Autodesk Inventor part; units mm, degrees
ref_plane "Work Plane1" through (-56.3599, 0, 22) normal (0, 0, -1) x (-1, 0, 0)
ref_plane "YZ Plane" through (0, 0, 0) normal (1, 0, 0) x (0, 1, 0)
ref_plane "XZ Plane" through (0, 0, 0) normal (0, 1, 0) x (-1, 0, 0)
ref_plane "Work Plane1" through (-56.3599, 0, 22) normal (0, 0, -1) x (-1, 0, 0)
sketch "Sketch1" plane through (-56.3599, 0, 22) normal (0, 0, -1) x (-1, 0, 0)
  line L0 (-4.0299, -0.3538) -> (-2.2322, 1.4439) construction
  arc A0 (-1.4439, 2.2322) -> (-2.2322, 1.4439) centre (-0.9299, 0.9299) ccw construction
  line L1 (-1.4439, 2.2322) -> (0.3538, 4.0299) construction
  line L2 (-37.8299, 42.8299) -> (-37.8299, 37.8299) construction
  line L3 (-37.8299, 37.8299) -> (-42.9208, 37.8299) construction
  line L4 (-37.8299, 42.2137) -> (-37.8299, 45.8299) construction
  line L5 (-37.8299, 45.8299) -> (-4.0299, 45.8299) construction
  line L6 (-4.0299, 45.8299) -> (-4.0299, 42.2137) construction
  line L7 (-4.0299, 4.0299) -> (0.3538, 4.0299)
  circle A1 centre (-20.9299, 20.9299) radius 17.5
  line L8 (-20.9299, 58.9723) -> (17.1124, 20.9299) construction
  line L9 (17.1124, 20.9299) -> (-20.9299, -17.1124) construction
  line L10 (-20.9299, -17.1124) -> (-58.9723, 20.9299) construction
  line L11 (-58.9723, 20.9299) -> (-20.9299, 58.9723) construction
  line L12 (-20.9299, 58.9723) -> (-20.9299, -17.1124) construction
  line L13 (17.1124, 20.9299) -> (-58.9723, 20.9299) construction
  line L14 (-20.9299, 58.9723) -> (32.8701, 58.9723) construction
  line L15 (-43.4299, 43.4299) -> (1.5701, 43.4299) construction
  line L16 (1.5701, 43.4299) -> (1.5701, -1.5701) construction
  line L17 (1.5701, -1.5701) -> (-43.4299, -1.5701) construction
  line L18 (-43.4299, -1.5701) -> (-43.4299, 43.4299) construction
  line L19 (-43.4299, 43.4299) -> (1.5701, -1.5701) construction
  line L20 (1.5701, 43.4299) -> (-43.4299, -1.5701) construction
  line L21 (-43.4299, 5.3876) -> (-43.4299, 36.4723)
  line L22 (-43.4299, 36.4723) -> (-36.4723, 43.4299)
  line L23 (-36.4723, 43.4299) -> (-5.3876, 43.4299)
  line L24 (-5.3876, 43.4299) -> (1.5701, 36.4723)
  line L25 (1.5701, 36.4723) -> (1.5701, 5.3876)
  line L26 (1.5701, 5.3876) -> (-5.3876, -1.5701)
  line L27 (-5.3876, -1.5701) -> (-36.4723, -1.5701)
  line L28 (-36.4723, -1.5701) -> (-43.4299, 5.3876)
  line L29 (-4.0299, 42.2137) -> (-37.8299, 42.2137)
  line L30 (-4.0299, -0.3538) -> (-4.0299, 4.0299)
  circle A2 centre (-20.9299, 20.9299) radius 1.5
  line L31 (-10.9299, 10.9299) -> (-30.9299, 10.9299) construction
  line L32 (-30.9299, 10.9299) -> (-30.9299, 30.9299) construction
  line L33 (-30.9299, 30.9299) -> (-10.9299, 30.9299) construction
  line L34 (-10.9299, 30.9299) -> (-10.9299, 10.9299) construction
  line L35 (-10.9299, 10.9299) -> (-30.9299, 30.9299) construction
  line L36 (-30.9299, 10.9299) -> (-10.9299, 30.9299) construction
  circle A3 centre (-30.9299, 30.9299) radius 1.4
  circle A4 centre (-30.9299, 10.9299) radius 1.4
  circle A5 centre (-10.9299, 10.9299) radius 1.4
  line L37 (-45.8299, 37.8299) -> (-42.0723, 37.8299) construction
  line L38 (-42.1723, 37.7299) -> (-45.8299, 37.7299)
  line L39 (-45.8299, 37.7299) -> (-45.8299, 4.1299)
  line L40 (-45.8299, 4.1299) -> (-42.1723, 4.1299)
  line L41 (-42.1723, 4.1299) -> (-42.1723, 37.7299)
  line L42 (-45.8299, 4.0299) -> (-42.0723, 4.0299) construction
  line L43 (-45.8299, 37.8299) -> (-42.0723, 37.8299)
  line L44 (-37.7299, 45.8299) -> (-4.1299, 45.8299)
  line L45 (-4.1299, 45.8299) -> (-4.1299, 42.1723)
  line L46 (-4.1299, 42.1723) -> (-37.7299, 42.1723)
  line L47 (-37.7299, 42.1723) -> (-37.7299, 45.8299)
  line L48 (0.4701, 37.8299) -> (0.4701, 4.0299) construction
  line L49 (0.4701, 4.0299) -> (3.9701, 4.0299) construction
  line L50 (3.9701, 37.8299) -> (3.9701, 4.0299) construction
  line L51 (0.4701, 37.8299) -> (3.9701, 37.8299) construction
  line L52 (-45.8299, -3.9701) -> (-4.0299, -3.9701) construction
  line L53 (0.3124, 37.7299) -> (3.9701, 37.7299)
  line L54 (3.9701, 37.7299) -> (3.9701, 4.1299)
  line L55 (3.9701, 4.1299) -> (0.3124, 4.1299)
  line L56 (0.3124, 4.1299) -> (0.3124, 37.7299)
  line L57 (-4.1713, -0.3538) -> (-37.7299, -0.3538)
  line L58 (-37.7299, -0.3538) -> (-37.7299, -3.9701)
  line L59 (-37.7299, -3.9701) -> (-4.1713, -3.9701)
  line L60 (-4.1713, -3.9701) -> (-4.1713, -0.3538)
  point P0 (-37.8299, 4.0299)
  dimension "d18" = 53.8
  dimension "d19" = 45
  dimension "d20" = 53.8
  dimension "d21" = 45
  dimension "d22" = 45
  dimension "d30" = 20
  dimension "d31" = 20
  dimension "d32" = 2.8
  dimension "d33" = 2.8
  dimension "d34" = 2.8
  dimension "d35" = 3
  dimension "d36" = 0.1
  dimension "d37" = 0.1
  dimension "d38" = 0.1
  dimension "d39" = 0.1
extrude "Extrusion1" add sketch "Sketch1" along normal blind 8 contours L30 L26 L57 L28 L41 L22 L46 L24 L56 L7 | L7 L26 L30 | L56 L24 L25 L26 | L26 L25 L24 L53 L54 L55 | L60 L59 L58 L57 L28 L27 L26 | L26 L27 L28 L57 | L46 L22 L29 L24 | L24 L29 L45 | L40 L39 L38 L22 L21 L28 | L28 L21 L22 L41 | L29 L22 L23 L24 | L24 L23 L22 L29 L47 L44 L45 | L47 L29 L22 | A1 | A2 | A3 | A4 | A5
sketch "Skizze4" plane through (-56.3599, 0, 14) normal (0, 0, -1) x (-1, 0, 0)
  line L0 (-37.7299, 42.1723) -> (-42.1723, 37.7299)
  line L1 (-42.1723, 37.7299) -> (-45.8299, 37.7299)
  line L2 (-45.8299, 37.7299) -> (-45.8299, 4.1299) construction
  line L3 (-45.8299, 4.1299) -> (-42.1723, 4.1299)
  line L4 (-42.1723, 4.1299) -> (-37.6885, -0.3538)
  line L5 (-37.6885, -0.3538) -> (-37.7299, -0.3538)
  line L6 (-37.7299, -0.3538) -> (-37.7299, -3.9701)
  line L7 (-37.7299, -3.9701) -> (-4.1713, -3.9701) construction
  line L8 (-4.1713, -3.9701) -> (-4.1713, -0.3538)
  line L9 (-4.1713, -0.3538) -> (0.3124, 4.1299)
  line L10 (0.3124, 4.1299) -> (3.9701, 4.1299)
  line L11 (3.9701, 4.1299) -> (3.9701, 37.7299) construction
  line L12 (3.9701, 37.7299) -> (0.3124, 37.7299)
  line L13 (0.3124, 37.7299) -> (-4.1299, 42.1723)
  line L14 (-4.1299, 42.1723) -> (-4.1299, 45.8299)
  line L15 (-4.1299, 45.8299) -> (-37.7299, 45.8299) construction
  line L16 (-37.7299, 45.8299) -> (-37.7299, 42.1723)
  line L17 (-37.9299, 46.0299) -> (-3.9299, 46.0299) construction
  line L18 (-3.9299, 46.0299) -> (-3.9299, 42.2551)
  line L19 (-3.9299, 42.2551) -> (0.3953, 37.9299)
  line L20 (0.3953, 37.9299) -> (4.1701, 37.9299)
  line L21 (4.1701, 37.9299) -> (4.1701, 3.9299) construction
  line L22 (4.1701, 3.9299) -> (0.3953, 3.9299)
  line L23 (0.3953, 3.9299) -> (-3.9713, -0.4367)
  line L24 (-3.9713, -0.4367) -> (-3.9713, -4.1701)
  line L25 (-3.9713, -4.1701) -> (-37.9299, -4.1701) construction
  line L26 (-37.9299, -4.1701) -> (-37.9299, -0.3953)
  line L27 (-37.9299, -0.3953) -> (-42.2551, 3.9299)
  line L28 (-42.2551, 3.9299) -> (-46.0299, 3.9299)
  line L29 (-46.0299, 3.9299) -> (-46.0299, 37.9299) construction
  line L30 (-46.0299, 37.9299) -> (-42.2551, 37.9299)
  line L31 (-42.2551, 37.9299) -> (-37.9299, 42.2551)
  line L32 (-37.9299, 42.2551) -> (-37.9299, 46.0299)
  line L33 (-45.8299, 37.7299) -> (-45.8299, 37.9299)
  line L34 (-4.1299, 45.8299) -> (-37.7299, 45.8299)
  line L35 (-37.7299, 45.8299) -> (-37.9299, 45.8299)
  line L36 (-4.1299, 45.8299) -> (-3.9299, 45.8299)
  line L37 (3.9701, 37.7299) -> (3.9701, 37.9299)
  line L38 (3.9701, 4.1299) -> (3.9701, 37.7299)
  line L39 (3.9701, 4.1299) -> (3.9701, 3.9299)
  line L40 (-4.1713, -3.9701) -> (-3.9713, -3.9701)
  line L41 (-37.7299, -3.9701) -> (-37.9299, -3.9701)
  line L42 (-45.8299, 4.1299) -> (-45.8299, 3.9299)
  point P0 (-56.3599, 0)
  dimension "d40" = 0.2
extrude "IM_offset" add sketch "Skizze4" against normal up to surface (8 mm away)
ref_plane "Arbeitsebene5" through (-35.4299, 3.9299, 22) normal (-1, 0, 0) x (0, 0, 1)
ref_plane "Arbeitsebene6" through (-18.4299, 20.9299, 22) normal (0, 1, 0) x (-1, 0, 0)
sketch "Skizze31" plane through (-56.3599, 0, 22) normal (0, 0, 1) x (1, 0, 0)
  line L0 (25.9049, 44.8899) -> (15.7949, 44.8899)
  spline S0 degree 3 poles (21.2744, 21.9194) (21.3357, 21.9462) (21.3936, 21.9718) (21.5033, 22.0154) (21.5491, 22.0289) (21.5827, 22.0289) (21.5892, 22.0276) (21.5935, 22.0247) knots 0.300335 0.300335 0.300335 0.300335 0.323424 0.323424 0.35266 0.35266 0.362351 0.362351 0.362351 0.362351
  line L1 (21.2744, 21.9194) -> (21.2744, 26.3899)
  line L2 (20.4254, 21.9194) -> (20.4254, 26.3899)
  line L3 (21.9714, 15.3899) -> (21.1087, 15.3899)
  line L4 (20.5911, 15.3899) -> (19.7285, 15.3899)
  line L5 (20.5999, 15.3899) -> (21.0999, 15.3899)
  line L6 (28.5999, 22.8289) -> (28.5999, 24.3299)
  line L7 (28.5999, 24.3299) -> (28.0999, 24.3299)
  line L8 (28.0999, 24.3299) -> (28.0999, 22.8289)
  line L9 (28.0999, 22.8289) -> (27.7114, 24.2788)
  line L10 (27.7114, 24.2788) -> (27.2285, 24.1494)
  line L11 (27.2285, 24.1494) -> (28.0911, 20.9299)
  line L12 (28.0911, 20.9299) -> (27.2285, 17.7105)
  line L13 (27.2285, 17.7105) -> (27.7114, 17.5811)
  line L14 (27.7114, 17.5811) -> (28.0999, 19.031)
  line L15 (28.0999, 19.031) -> (28.0999, 17.5299)
  line L16 (28.0999, 17.5299) -> (28.5999, 17.5299)
  line L17 (28.5999, 17.5299) -> (28.5999, 19.031)
  line L18 (28.5999, 19.031) -> (28.9884, 17.5811)
  line L19 (28.9884, 17.5811) -> (29.4714, 17.7105)
  line L20 (29.4714, 17.7105) -> (28.6087, 20.9299)
  line L21 (28.6087, 20.9299) -> (29.4714, 24.1494)
  line L22 (29.4714, 24.1494) -> (28.9884, 24.2788)
  line L23 (28.9884, 24.2788) -> (28.5999, 22.8289)
  circle A0 centre (28.3499, 20.9299) radius 1.35
  line L24 (3.9713, -3.9701) -> (37.9299, -3.9701)
  line L25 (37.9299, -3.9701) -> (37.9299, -0.3953)
  line L26 (37.9299, -0.3953) -> (42.2551, 3.9299)
  line L27 (42.2551, 3.9299) -> (45.8299, 3.9299)
  line L28 (45.8299, 3.9299) -> (45.8299, 37.9299)
  line L29 (45.8299, 37.9299) -> (42.2551, 37.9299)
  line L30 (42.2551, 37.9299) -> (37.9299, 42.2551)
  line L31 (37.9299, 42.2551) -> (37.9299, 45.8299)
  line L32 (37.9299, 45.8299) -> (3.9299, 45.8299)
  line L33 (3.9299, 45.8299) -> (3.9299, 42.2551)
  line L34 (3.9299, 42.2551) -> (-0.3953, 37.9299)
  line L35 (-0.3953, 37.9299) -> (-3.9701, 37.9299)
  line L36 (-3.9701, 37.9299) -> (-3.9701, 3.9299)
  line L37 (-3.9701, 3.9299) -> (-0.3953, 3.9299)
  line L38 (-0.3953, 3.9299) -> (3.9713, -0.4367)
  line L39 (3.9713, -0.4367) -> (3.9713, -3.9701)
  line L40 (45.8299, 37.9299) -> (45.8299, 3.9299)
  line L41 (20.8299, 20.4299) -> (45.8299, 20.4299)
  line L42 (45.8299, 20.4299) -> (45.8299, 21.4299)
  line L43 (45.8299, 21.4299) -> (20.8299, 21.4299)
  line L44 (20.8299, 21.4299) -> (20.8299, 20.4299)
  line L45 (20.8299, 20.4299) -> (45.8299, 21.4299) construction
  line L46 (45.8299, 20.4299) -> (20.8299, 21.4299) construction
  line L47 (45.8299, 30.4299) -> (20.8299, 30.4299)
  line L48 (20.8299, 30.4299) -> (20.8299, 27.4299)
  line L49 (20.8299, 27.4299) -> (45.8299, 27.4299)
  line L50 (45.8299, 27.4299) -> (45.8299, 30.4299)
  line L51 (45.8299, 14.4299) -> (20.8299, 14.4299)
  line L52 (20.8299, 14.4299) -> (20.8299, 11.4299)
  line L53 (20.8299, 11.4299) -> (45.8299, 11.4299)
  line L54 (45.8299, 11.4299) -> (45.8299, 14.4299)
  circle A1 centre (20.8299, 20.9299) radius 1.5
  point P0 (56.3599, 0)
  point P1 (33.3299, 20.9299)
  point P2 (45.8299, 11.4299)
  point P3 (27.0959, 20.4299)
  point P4 (29.6039, 20.4299)
  point P5 (29.6039, 21.4299)
  point P6 (27.0959, 21.4299)
  point P7 (22.2441, 21.4299)
  point P8 (22.2441, 20.4299)
  point P9 (45.8299, 27.4299)
  dimension "d181" = 2.7
  dimension "d182" = 1
  dimension "d183" = 3
  dimension "d184" = 3
  dimension "d185" = 25
  dimension "d186" = 0
  dimension "d187" = 3
  dimension "d197" = 6
  dimension "d198" = 6
extrude "Extrusion26" cut sketch "Skizze31" against normal blind 10 contours A0 L43 L21 | L21 L43 L11 A0 | L43 A0 L41 L20 L21 | L21 L20 L41 L12 L11 L43 | L43 L28 L41 A0 | L11 L43 A0 | L11 L12 L41 A0 L43 | A0 L41 A1 L43 | L41 A0 L20 | L20 A0 L12 L41 | L49 L48 L47 L28 | L41 L12 A0 | A1 L41 L44 L43 | L43 L44 L41 A1 | L28 L53 L52 L51
sketch "Skizze32" plane through (-35.5299, -3.9701, 22) normal (0, -1, 0) x (1, 0, 0)
  line L0 (8.774, 0) -> (8.774, -8)
  line L1 (6.266, 0) -> (6.266, -8)
  line L2 (-16.8586, 0) -> (17.1, 0)
  line L3 (-16.8586, -8) -> (-16.8586, 0)
  line L4 (-16.8586, -8) -> (17.1, -8)
  line L5 (17.1, -8) -> (17.1, 0)
  circle A0 centre (13.0607, -4) radius 0.7419
  point P0 (35.5299, -22)
hole "Bohrung2" at (-22.4692, -3.9701, 18) direction (0, 1, 0) diameter 2.8 depth 35 tip angle 118 counterbore diameter 6.5 counterbore depth 16
properties part number "20_Cube_Insert_2D_Galvo_Fiberlaunch_v3"
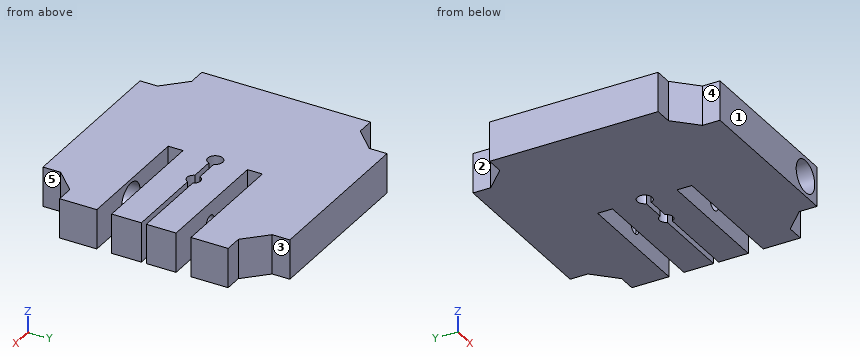
Design review of the part built by this model. Coordinates are the model's own, in mm. Face numbers are marked on the shaded views. A direction names the side the tool comes from. Coordinates: 2 decimals unless noted, no trailing zeros. Loops run counter-clockwise (first coordinate to the right, second up) from the corner with the lowest first, then second, coordinate; pieces in that order, holes last.
Q1. We need section C-C on x = -55.5. State the section outline as (y, z) points, and give its area (3 significant figures).
Reported:
outline: (2.67, 14) - (39.19, 14) - (39.19, 22) - (2.67, 22) - close
area: 292 mm2
Q2. We need section B-B on y = 41. State the section outline as (x, z) points, and give its area (3 significant figures).
Reported:
outline: (-53.69, 14) - (-17.17, 14) - (-17.17, 22) - (-53.69, 22) - close
area: 292 mm2
Q3. Tool access review of the marked faces 1, 2, 3, 4 and 5: name each direction out of +Z, -Z, +X, -X, +Y, -Y from which nothing blocks a thin tool from reaching the whole face with its end or side.
Reported:
face 1: +Z, -Z, +X, -X, -Y
face 2: +Z, -Z, -X, +Y
face 3: +Z, -Z, +X, +Y
face 4: +Z, -Z, -X, -Y
face 5: +Z, -Z, +X, -Y
Q4. For pin 1 (3 mm diameter, centred on x = -22.47, z = 18, fed in from -Y); pin 2 (1.8 mm diameter, centred on y = 44, z = 18, fed in from +X); pin 3 (1.8 mm diameter, centred on x = -35.53, y = 20.93, fed in from -Z); pin 4 (3 mm diameter, centred on x = -59, z = 19, fed in from +Y), all flat-tipped, find the tip position at first contact; note any pin that passes through.
Reported:
pin 1: stops at y = 14.43
pin 2: stops at x = -18.43
pin 3: passes through
pin 4: stops at y = 37.93
Q5. To check wall thickness, follow line 1 (Y direction, x = -14, z = 21.5); line 2 (Y direction, x = -19.5, z = 20.5); line 3 (X direction, y = 23.3, z = 18). State the ranges of each line that lie inside material, in increasing order.
Reported:
line 1: y = 3.93 to 11.43, 14.43 to 20.43, 21.43 to 27.43, 30.43 to 37.93
line 2: y = -3.97 to 11.43, 14.43 to 20.43, 21.43 to 27.43, 30.43 to 45.83
line 3: x = -60.33 to -23.87, -21.07 to -10.53
Q6. We need section A-A on y = 7. State the section outline as (x, z) points.
Reported:
outline: (-60.33, 14) - (-10.53, 14) - (-10.53, 22) - (-60.33, 22) - close; hole circle Ø6.5 at (-22.47, 18)
